```python
from build123d import *

# Parameters (mm, degrees)
SHELL1_T = -2.54


with BuildPart() as part:
    # Sketch1 → Revolve1 (revolve)
    with BuildSketch(Plane.XY, mode=Mode.PRIVATE) as revolve1_sk:
        with BuildLine():
            Line((-49.53, 0), (-49.53, 130.556))
            ThreePointArc((-49.53, 130.556), (-38.537049964, 192.463531829), (-6.902305408, 246.801643541))
            ThreePointArc((-6.902305408, 246.801643541), (-3.803659553, 249.161559344), (0, 250))
            Line((0, 250), (0, 0))
            Line((0, 0), (-49.53, 0))
        make_face()
    revolve(revolve1_sk.sketch.rotate(Axis((0, 255.455794576, 0), (0, -1, 0)), 270), axis=Axis((0, 255.455794576, 0), (0, -1, 0)))

    # Shell1
    shell1_openings = [part.faces().sort_by_distance(p)[0] for p in [
        (0, 0, 0),
    ]]
    offset(amount=SHELL1_T, openings=shell1_openings, kind=Kind.INTERSECTION)


solid = part.part
```
Part model, mm, in its own coordinate system. Give positions to 0.01 mm unless a question says otherwise; leave off trailing zeros. Order: outer loops, then holes, each group sorted by start corner. A loop starts at its lowest first (then second) coordinate and runs counter-clockwise, first axis right, second up. Notation, with made-up numbers: M 19.25,-15 L 69.25,-15 A28 ccw 69.25,23 Z; hole C 8,57 d2. An arc over 180 degrees is marked long. Use a Markdown table: item, result. Add a question column.
(1) Drop flat-ended pins along their axis: P1, Ø12, axis at y = 194, z = 8.5, coming from the -X side; P2, Ø4, axis at x = 18, z = 14.5, coming from the +Y side; P3, Ø8, axis at x = -2.5, y = 62, coming from the -Z side; P4, Ø10, axis at y = 80, z = -11.5, coming from the +X side. Give the stop position or say it passes through.
(2) Probe line 1 along X through (y, z) = (67, 0); line 2 along X through (y, z) = (85.5, 40); line 3 along Z through (x, y) = (27, 76). List the from-to ranges inside material, lowest first. Write a range as [from, to].
(3) Mould opens along Z. For faces 1 (the face through (44, 0, -18)), 2 (the face through (-14.88, 66.19, 47.24)), 3 (the face through (45.87, 66.19, -10.19)) say: +Z half, -Z half, draft (parallel to the pull), parting line (faces both ways), or undercut.
(4) Saw through at A-A, the plane y = 126. Give the cut face in (x, z), and give its area (3 significant figures).
Answer key:
| question | item | result |
|---|---|---|
| 1 | P1 | x = -39.47 |
| 1 | P2 | y = 227.57 |
| 1 | P3 | z = -49.53 |
| 1 | P4 | x = 49.1 |
| 2 | line 1 | [-49.53, -46.99], [46.99, 49.53] |
| 2 | line 2 | [-29.21, -24.66], [24.66, 29.21] |
| 2 | line 3 | [-41.52, -38.46], [38.46, 41.52] |
| 3 | face 1 | draft |
| 3 | face 2 | parting line |
| 3 | face 3 | undercut |
| 4 | outline | C 0,0 d99.06; hole C 0,0 d93.98 |
| 4 | area | 770 mm^2 |
